Autodesk Inventor part; units mm, degrees
ref_plane "YZ Plane" through (0, 0, 0) normal (1, 0, 0) x (0, 1, 0)
ref_plane "XZ Plane" through (0, 0, 0) normal (0, 1, 0) x (-1, 0, 0)
ref_plane "XY Plane" through (0, 0, 0) normal (0, 0, 1) x (1, 0, 0)
sketch "Sketch1" plane through (0, 0, 0) normal (1, 0, 0) x (0, 1, 0)
  circle A0 centre (0, 0) radius 12.5095
  dimension "d0" = 25.019
extrude "Extrusion1" add sketch "Sketch1" along normal blind 7.747
sketch "Sketch3" plane through (7.747, 0, 0) normal (1, 0, 0) x (0, 0, -1)
  circle A0 centre (0, 0) radius 12.5095
  circle A1 centre (0, 0) radius 8.763
  dimension "d3" = 17.526
extrude "Extrusion2" add sketch "Sketch3" along normal blind 8.89 contours A1
sketch "Sketch4" plane through (7.747, 0, 0) normal (1, 0, 0) x (0, 0, -1)
  circle A0 centre (0, 0) radius 8.763
  circle A1 centre (0, 0) radius 6.7818
  dimension "d26" = 6.7818
extrude "Extrusion3" cut sketch "Sketch4" along normal blind 1.397
sketch "Sketch5" plane through (16.637, 0, 0) normal (1, 0, 0) x (0, 0, -1)
  circle A0 centre (0, 0) radius 8.763
hole "Hole1" at (16.637, 0, 0) direction (-1, 0, 0) diameter 9.525 end through all
sketch "Sketch6" plane through (0, 0, 0) normal (-1, 0, 0) x (0, 0, 1)
  circle A0 centre (0, 0) radius 4.7625
hole "Hole2" at (0, 0, 0) direction (1, 0, 0) diameter 23.114 depth 6.8072
sketch "Sketch7" plane through (16.637, 0, 0) normal (1, 0, 0) x (0, 0, -1)
  circle A0 centre (0, 0) radius 8.763
  arc A1 (6.3049, -2.5147) -> (8.3872, -2.5234) centre (7.3744, 4.2693) ccw
  arc A2 (8.3872, -2.5234) -> (8.5753, -1.7828) centre (0, 0) ccw
  arc A3 (8.5753, -1.7828) -> (6.741, -0.7972) centre (4.445, -7.2699) ccw
  arc A4 (6.741, -0.7972) -> (6.7848, -0.2067) centre (0, 0) ccw
  arc A5 (6.7848, -0.2067) -> (8.7445, 0.4974) centre (5.4695, 6.534) ccw
  arc A6 (8.7445, 0.4974) -> (8.6679, 1.2576) centre (0, 0) ccw
  arc A7 (8.6679, 1.2576) -> (6.6071, 1.5564) centre (6.6633, -5.3112) ccw
  arc A8 (6.6071, 1.5564) -> (6.4463, 2.1263) centre (0, 0) ccw
  arc A9 (6.4463, 2.1263) -> (8.047, 3.4581) centre (2.9049, 8.0107) ccw
  arc A10 (8.047, 3.4581) -> (7.715, 4.1463) centre (0, 0) ccw
  arc A11 (7.715, 4.1463) -> (5.6763, 3.7223) centre (8.078, -2.7119) ccw
  arc A12 (5.6763, 3.7223) -> (5.3303, 4.2029) centre (0, 0) ccw
  arc A13 (5.3303, 4.2029) -> (6.379, 6.0018) centre (-0.0101, 8.5211) ccw
  arc A14 (6.379, 6.0018) -> (5.8316, 6.535) centre (0, 0) ccw
  arc A15 (5.8316, 6.535) -> (4.0609, 5.4392) centre (8.5184, 0.2145) ccw
  arc A16 (4.0609, 5.4392) -> (3.5714, 5.7725) centre (0, 0) ccw
  arc A17 (3.5714, 5.7725) -> (3.9415, 7.8216) centre (-2.9239, 8.0037) ccw
  arc A18 (3.9415, 7.8216) -> (3.2448, 8.1354) centre (0, 0) ccw
  arc A19 (3.2448, 8.1354) -> (1.9557, 6.5001) centre (7.9313, 3.115) ccw
  arc A20 (1.9557, 6.5001) -> (1.3817, 6.6458) centre (0, 0) ccw
  arc A21 (1.3817, 6.6458) -> (1.0287, 8.698) centre (-5.485, 6.521) ccw
  arc A22 (1.0287, 8.698) -> (0.2667, 8.7546) centre (0, 0) ccw
  arc A23 (0.2667, 8.7546) -> (-0.3854, 6.777) centre (6.3876, 5.6398) ccw
  arc A24 (-0.3854, 6.777) -> (-0.9746, 6.7176) centre (0, 0) ccw
  arc A25 (-0.9746, 6.7176) -> (-2.0083, 8.5253) centre (-7.3845, 4.2518) ccw
  arc A26 (-2.0083, 8.5253) -> (-2.7436, 8.3178) centre (0, 0) ccw
  arc A27 (-2.7436, 8.3178) -> (-2.6801, 6.2364) centre (4.0734, 7.4844) ccw
  arc A28 (-2.6801, 6.2364) -> (-3.2134, 5.9791) centre (0, 0) ccw
  arc A29 (-3.2134, 5.9791) -> (-4.803, 7.3243) centre (-8.3934, 1.4697) ccw
  arc A30 (-4.803, 7.3243) -> (-5.423, 6.8778) centre (0, 0) ccw
  arc A31 (-5.423, 6.8778) -> (-4.6514, 4.9437) centre (1.268, 8.4262) ccw
  arc A32 (-4.6514, 4.9437) -> (-5.0646, 4.5195) centre (0, 0) ccw
  arc A33 (-5.0646, 4.5195) -> (-7.0184, 5.2399) centre (-8.3899, -1.4896) ccw
  arc A34 (-7.0184, 5.2399) -> (-7.4483, 4.6082) centre (0, 0) ccw
  arc A35 (-7.4483, 4.6082) -> (-6.0618, 3.0547) centre (-1.6904, 8.3517) ccw
  arc A36 (-6.0618, 3.0547) -> (-6.3049, 2.5147) centre (0, 0) ccw
  arc A37 (-6.3049, 2.5147) -> (-8.3872, 2.5234) centre (-7.3744, -4.2693) ccw
  arc A38 (-8.3872, 2.5234) -> (-8.5753, 1.7828) centre (0, 0) ccw
  arc A39 (-8.5753, 1.7828) -> (-6.741, 0.7972) centre (-4.445, 7.2699) ccw
  arc A40 (-6.741, 0.7972) -> (-6.7848, 0.2067) centre (0, 0) ccw
  arc A41 (-6.7848, 0.2067) -> (-8.7445, -0.4974) centre (-5.4695, -6.534) ccw
  arc A42 (-8.7445, -0.4974) -> (-8.6679, -1.2576) centre (0, 0) ccw
  arc A43 (-8.6679, -1.2576) -> (-6.6071, -1.5564) centre (-6.6633, 5.3112) ccw
  arc A44 (-6.6071, -1.5564) -> (-6.4463, -2.1263) centre (0, 0) ccw
  arc A45 (-6.4463, -2.1263) -> (-8.047, -3.4581) centre (-2.9049, -8.0107) ccw
  arc A46 (-8.047, -3.4581) -> (-7.715, -4.1463) centre (0, 0) ccw
  arc A47 (-7.715, -4.1463) -> (-5.6763, -3.7223) centre (-8.078, 2.7119) ccw
  arc A48 (-5.6763, -3.7223) -> (-5.3303, -4.2029) centre (0, 0) ccw
  arc A49 (-5.3303, -4.2029) -> (-6.379, -6.0018) centre (0.0101, -8.5211) ccw
  arc A50 (-6.379, -6.0018) -> (-5.8316, -6.535) centre (0, 0) ccw
  arc A51 (-5.8316, -6.535) -> (-4.0609, -5.4392) centre (-8.5184, -0.2145) ccw
  arc A52 (-4.0609, -5.4392) -> (-3.5714, -5.7725) centre (0, 0) ccw
  arc A53 (-3.5714, -5.7725) -> (-3.9415, -7.8216) centre (2.9239, -8.0037) ccw
  arc A54 (-3.9415, -7.8216) -> (-3.2448, -8.1354) centre (0, 0) ccw
  arc A55 (-3.2448, -8.1354) -> (-1.9557, -6.5001) centre (-7.9313, -3.115) ccw
  arc A56 (-1.9557, -6.5001) -> (-1.3817, -6.6458) centre (0, 0) ccw
  arc A57 (-1.3817, -6.6458) -> (-1.0287, -8.698) centre (5.485, -6.521) ccw
  arc A58 (-1.0287, -8.698) -> (-0.2667, -8.7546) centre (0, 0) ccw
  arc A59 (-0.2667, -8.7546) -> (0.3854, -6.777) centre (-6.3876, -5.6398) ccw
  arc A60 (0.3854, -6.777) -> (0.9746, -6.7176) centre (0, 0) ccw
  arc A61 (0.9746, -6.7176) -> (2.0083, -8.5253) centre (7.3845, -4.2518) ccw
  arc A62 (2.0083, -8.5253) -> (2.7436, -8.3178) centre (0, 0) ccw
  arc A63 (2.7436, -8.3178) -> (2.6801, -6.2364) centre (-4.0734, -7.4844) ccw
  arc A64 (2.6801, -6.2364) -> (3.2134, -5.9791) centre (0, 0) ccw
  arc A65 (3.2134, -5.9791) -> (4.803, -7.3243) centre (8.3934, -1.4697) ccw
  arc A66 (4.803, -7.3243) -> (5.423, -6.8778) centre (0, 0) ccw
  arc A67 (5.423, -6.8778) -> (4.6514, -4.9437) centre (-1.268, -8.4262) ccw
  arc A68 (4.6514, -4.9437) -> (5.0646, -4.5195) centre (0, 0) ccw
  arc A69 (5.0646, -4.5195) -> (7.0184, -5.2399) centre (8.3899, 1.4896) ccw
  arc A70 (7.0184, -5.2399) -> (7.4483, -4.6082) centre (0, 0) ccw
  arc A71 (7.4483, -4.6082) -> (6.0618, -3.0547) centre (1.6904, -8.3517) ccw
  arc A72 (6.0618, -3.0547) -> (6.3049, -2.5147) centre (0, 0) ccw
extrude "Extrusion4" cut sketch "Sketch7" against normal up to surface (7.493 mm away)
properties part number "Clutch Gear" material "Stainless Steel, 440C"
Can you work these out from the model? Positions are in its coordinate system, mm. A direction names the side the tool comes from. Coordinates: 2 decimals unless noted, no trailing zeros. Loops run counter-clockwise (first coordinate to the right, second up) from the corner with the lowest first, then second, coordinate; pieces in that order, holes last. Notation, with made-up numbers: M 23,58 L 48,58 A4 cw 48,64 Z; hole C 17,36 d11. An arc over 180 degrees is marked long. Answer as CSV lines item,"result". Start each with the question number.
1. If I drill on probe 1 along Y at (x, z) = (11, -1); probe 2 along Y at (x, z) = (12.25, 7.75); probe 3 along Z at (x, y) = (2.25, 0), over which ranges is the centre line in solid material (lowest first)? Write a range as [from, to].
2. Suppose I cut it at A-A, the plane x = 1.75. List the corners of the cut face in (y, z) for me.
3. Suppose I cut it at B-B, the plane z = 9.75. List the corners of the cut face in (x, y) for me, plus the area to 3 significant figures.
4. For faces 4 (the face through (12.943, 2.722, -7.286)), 5 (the face through (12.94, 7.8, 0.13)), 6 (the face through (12.94, 1.23, 7.71)), which set-ups out of +Z, -Z, +X, -X, +Y, -Y let a thin tool reach every point of the face, with its end or its side?
5. Thinking about a two-plate mould opening in Z: for faces 1 (the face through (8.436, -2.037, -6.469)), 2 (the face through (12.943, -3.79, -6.824)), 3 (the face through (12.94, -7.38, 2.55)), which applies, +Z half, -Z half, draft (parallel to the pull), parting line (faces both ways), or undercut?
6. For pin 1 Ø1 at (y, z) = (6, 2.5) entering from -X; pin 2 Ø6 at (x, z) = (12.5, 8) entering from +Y; pin 3 Ø3 at (x, y) = (9, -3) entering from -Z, each with a flat end and sliding along its axis, tell me the tip position at first contact or that it passes through.
Output:
1,probe 1,"y = [-6.78, -4.66], [4.66, 8.7]"
1,probe 2,"y = [-4.08, -3.14], [-1.47, -0.06], [1.25, 2.59]"
1,probe 3,"z = [-12.51, -11.56], [11.56, 12.51]"
2,outline,"C 0,0 d25.02; hole C 0,0 d23.11"
3,outline,"M 0,-7.84 L 7.75,-7.84 L 7.75,7.84 L 0,7.84 L 0,6.2 L 6.81,6.2 L 6.81,-6.2 L 0,-6.2 Z"
3,area,"37.0 mm^2"
4,face 4,"-Z, +X"
4,face 5,"+X, +Y"
4,face 6,"+Z, +X"
5,face 1,"parting line"
5,face 2,"-Z half"
5,face 3,"undercut"
6,pin 1,"stops at x = 6.81"
6,pin 2,"stops at y = 7.19"
6,pin 3,"stops at z = -12.32"
